Here's the drawing with two shaded views (mm, measured from the low corner). I have some questions. Round coordinates to 2 decimals unless told otherwise and drop trailing zeros. Order: outer loops, then holes, each group sorted by start corner. A loop starts at its lowest first (then second) coordinate and runs counter-clockwise, first axis right, second up. Notation, with made-up numbers: M 78.25,2 L 121.25,2 A17 cw 121.25,6 Z; hole C 61,-26.5 d1. An arc over 180 degrees is marked long. One line per question, with ' | ' between items.
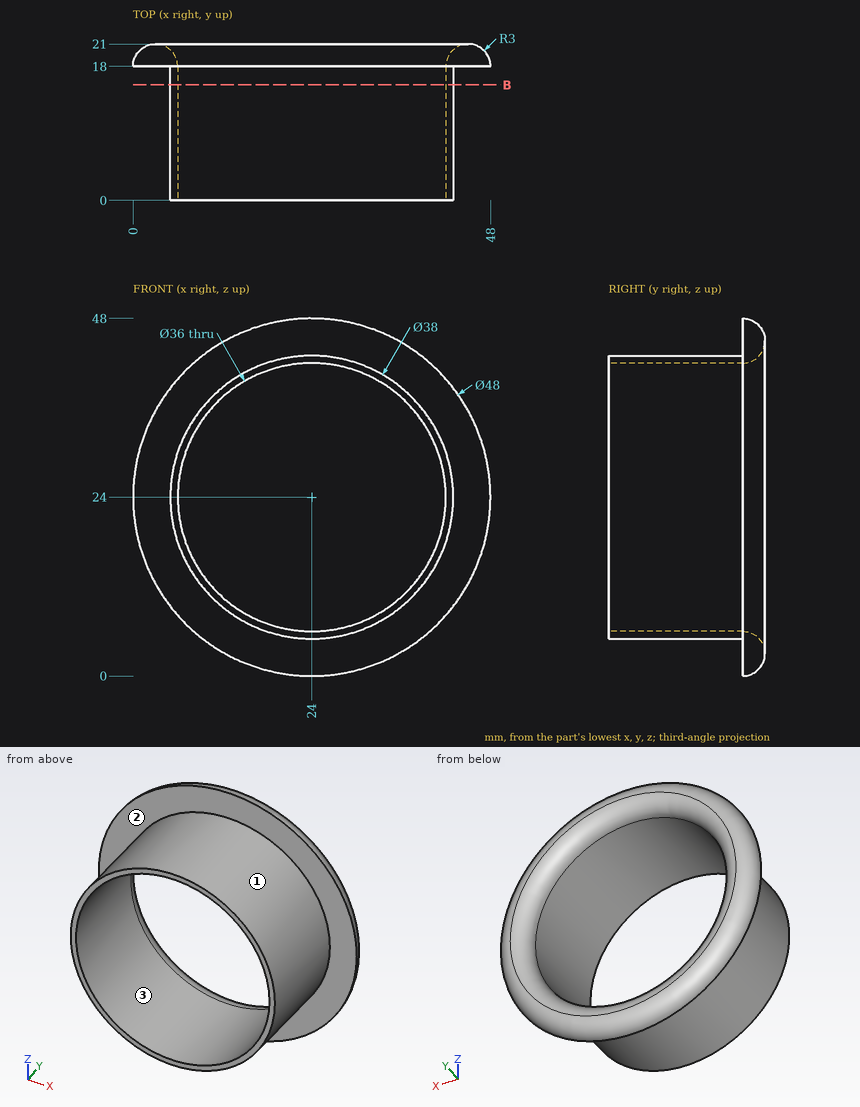
(1) Will these pins go through, and if not, where does the flat tip stop? pin 1 Ø1 at (y, z) = (18, 39) entering from +X; pin 2 Ø1.5 at (x, z) = (7.5, 21) entering from +Y; pin 3 Ø8 at (x, z) = (10, 15.5) entering from +Y; pin 4 Ø10 at (x, y) = (13, 11.5) entering from -Z.
Final values:
pin 1: x = 43.12 | pin 2: through | pin 3: y = 20.93 | pin 4: z = 5.97
(2) Please list where these lines run through material, in increasing order: probe 1 along Z at (x, y) = (24, 6.75); probe 2 along Y at (x, z) = (43, 14.5); probe 3 along Z at (x, y) = (40.5, 2). Write a range as [from, to].
Final values:
probe 1: [5, 6], [42, 43] | probe 2: [18, 20.99] | probe 3: [14.58, 16.81], [31.19, 33.42]
(3) If we section it at B-B on y = 15.5: Please give me the cut outline in (x, z).
Final values:
outline: C 24,24 d38; hole C 24,24 d36
(4) Thinking about a two-plate mould opening in X: for the marked faces 1, 2 and 3, which applies, released by +X, released by -X, zero draft, split by the parting line, or undercut?
Final values:
face 1: split by the parting line | face 2: zero draft | face 3: undercut
